Input: part model. Units: mm. Frame: model coordinates. Coordinates: 2 decimals unless noted, no trailing zeros. Write each loop counter-clockwise with the first axis right and the second up, starting at its lowest first coordinate (ties: lowest second). Pieces come first, ordered by that corner, then holes.
from build123d import *

# Parameters (mm, degrees)
F1_DEPTH = 2.54
F2_R     = 12.7
F3_DEPTH = 2.541
F2_R_2   = 7.9375
F4_DEPTH = 25.4
F5_R     = 2.5527
F6_DEPTH = 25.4


# Not quite as in the source:
# - a feature names something its author has since deleted; it is built from what else it names


with BuildPart() as f1:
    # F0 (on Right) → F1 (new body)
    with BuildSketch(Plane.YZ):
        with BuildLine():
            ThreePointArc((0, 6.35), (1.8598719395, 1.8598719395), (6.35, 0))
            Line((6.35, 0), (165.1, 0))
            Line((165.1, 0), (165.1, 88.9))
            Line((165.1, 88.9), (6.35, 88.9))
            ThreePointArc((6.35, 88.9), (1.8598719395, 87.0401280605), (0, 82.55))
            Line((0, 82.55), (0, 6.35))
        make_face()
    extrude(amount=F1_DEPTH)

    # F2 (on face) → F3 (cut, through all)
    with BuildSketch(Plane.YZ.offset(2.54)):
        with Locations((38.1, 63.5)):
            Circle(F2_R)
    extrude(amount=-F3_DEPTH, mode=Mode.SUBTRACT)

    # F2 (on face) → F4 (cut)
    with BuildSketch(Plane.YZ.offset(2.54)):
        with Locations((38.1, 63.5)):
            Circle(F2_R)
        with Locations((149.225, 60.325)):
            Circle(F2_R_2)
    extrude(amount=-F4_DEPTH, mode=Mode.SUBTRACT)

    # F5 (on face) → F6 (cut)
    with BuildSketch(Plane.YZ.offset(2.54)):
        with Locations((5.08, 65.024)):
            Circle(F5_R)
        with Locations((71.12, 65.024)):
            Circle(F5_R)
    extrude(amount=-F6_DEPTH, mode=Mode.SUBTRACT)


solid = f1.part
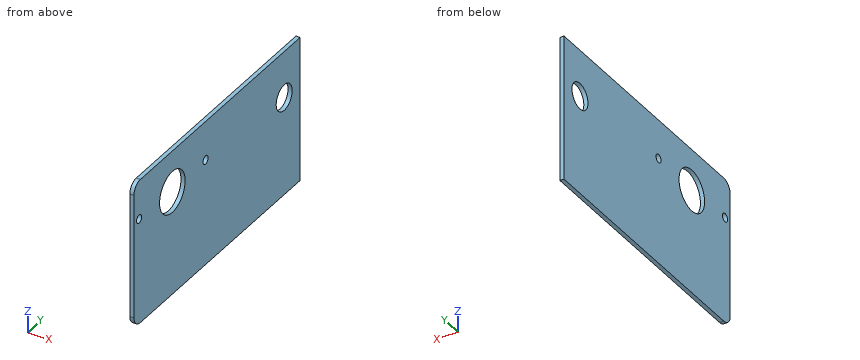
Item 1: Material intervals for line 1 (Z direction, x = 1.5, y = 38.1); line 2 (Y direction, x = 1.4, z = 62); line 3 (Z direction, x = 0.85, y = 71.12), sorted ascending.
Item 2: Section query B-B, the plane x = 0.4. State how many separate pieces and enclosed holes the cut face has, then the cut area to 3 significant figures.
Item 3: Section query A-A, the plane y = 38.1. Return loops of the section in (x, z).
Item 4: Section query C-C, the plane y = 71.12. Return loops of the section in (x, z).
The answers:
1. line 1: z = 0 to 50.8, 76.2 to 88.9
1. line 2: y = 0 to 25.49, 50.71 to 141.47, 156.98 to 165.1
1. line 3: z = 0 to 62.47, 67.58 to 88.9
2. separate pieces: 1
2. enclosed holes: 4
2. area: 13,900 mm2
3. outline: (0, 0) - (2.54, 0) - (2.54, 50.8) - (0, 50.8) - close; (0, 76.2) - (2.54, 76.2) - (2.54, 88.9) - (0, 88.9) - close
4. outline: (0, 0) - (2.54, 0) - (2.54, 62.47) - (0, 62.47) - close; (0, 67.58) - (2.54, 67.58) - (2.54, 88.9) - (0, 88.9) - close
